Verification items for this drawing (mm, ordinates from the low corner). A direction names the side the tool comes from. Round coordinates to 2 decimals unless told otherwise and drop trailing zeros. Order: outer loops, then holes, each group sorted by start corner. A loop starts at its lowest first (then second) coordinate and runs counter-clockwise, first axis right, second up. Notation, with made-up numbers: (8, 23.25) - (12, 23.25) arc R35 cw to (12, 61.25) - close; hole circle Ø1 at (11.25, -9). An arc over 180 degrees is marked (long way). Return JSON: item names as keys, results as strings. Group by question number.
Q1. Material ranges on line 1 along X through (y, z) = (37.5, 45); line 2 along Z through (x, y) = (107, 40.5) (1 decimal); line 3 along Y through (x, z) = (88, 25.5) (1 decimal), recorded low to high.
Q2. Sectioned sample at D-D, the plane z = 35. Record the cut outline in (x, y).
Q3. Sectioned sample at B-B, the plane y = 28. Record the cut outline in (x, z).
Q4. Gauge pin test, flat ends, axial feed: pin 1 Ø12 at (x, y) = (36.5, 28) entering from -Z (1 decimal); pin 2 Ø3 at (y, z) = (20, 17) entering from -X; pin 3 Ø2 at (x, z) = (91.5, 18) entering from +Y. Record the tip position at first contact, or that the pin passes through.
Q5. Tool access check on the marked faces 1 and 2. Record the directions out of +Z, -Z, +X, -X, +Y, -Y that give a thin tool (end or side, any length) a straight path to the whole face; none if there is none.
Q6. Sectioned sample at C-C, the plane x = 84. Record the cut outline in (y, z), then the cut area to 3 significant figures.
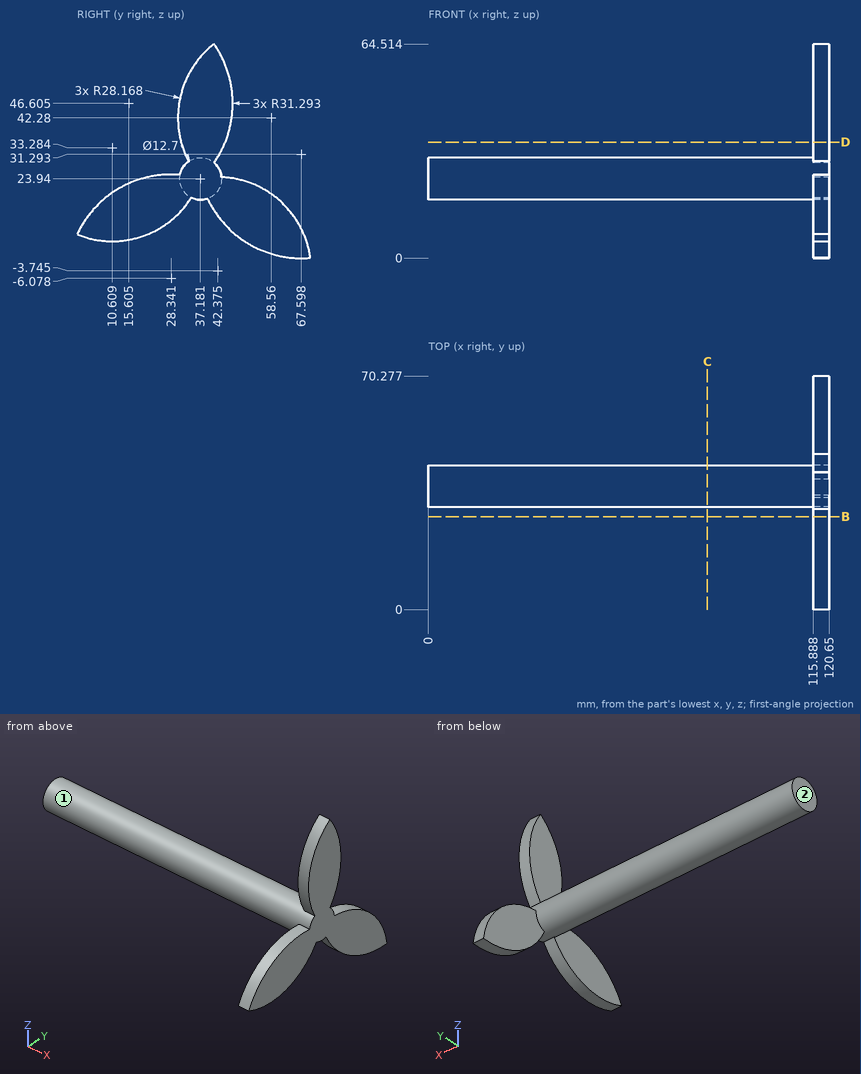
Reply:
{
 "1": {"line 1": "115.89 to 120.65", "line 2": "18.5 to 29.4", "line 3": "31 to 43.3"},
 "2": {"outline": "(115.89, 31.35) - (120.65, 31.35) - (120.65, 44.67) - (115.89, 44.67) - close"},
 "3": {"outline": "(115.89, 11.13) - (120.65, 11.13) - (120.65, 25.21) - (115.89, 25.21) - close"},
 "4": {"pin 1": "z = 18.4", "pin 2": "x = 115.89", "pin 3": "y = 41.17"},
 "5": {"face 1": "-X", "face 2": "+Z, -Z, -X, +Y, -Y"},
 "6": {"outline": "circle Ø12.7 at (37.18, 23.94)", "area": "127 mm^2"}
}
